Autodesk Inventor part; units mm, degrees
ref_plane "YZ Plane" through (0, 0, 0) normal (1, 0, 0) x (0, 1, 0)
ref_plane "XZ Plane" through (0, 0, 0) normal (0, 1, 0) x (-1, 0, 0)
ref_plane "XY Plane" through (0, 0, 0) normal (0, 0, 1) x (1, 0, 0)
sketch "Sketch1" plane through (0, 0, 0) normal (0, 0, 1) x (1, 0, 0)
  circle A0 centre (0, 0) radius 5
  line L0 (0, 7.8889) -> (6.832, 3.9445)
  line L1 (6.832, 3.9445) -> (6.832, -3.9445)
  line L2 (6.832, -3.9445) -> (0, -7.8889)
  line L3 (0, -7.8889) -> (-6.832, -3.9445)
  line L4 (-6.832, -3.9445) -> (-6.832, 3.9445)
  line L5 (-6.832, 3.9445) -> (0, 7.8889)
  dimension "d0" = 10
extrude "Extrusion1" add sketch "Sketch1" along normal blind 5.08
thread "Thread1"
properties part number "Nut"
Design review of the part built by this model. Coordinates are the model's own, in mm. Give positions to 0.01 mm unless a question says otherwise; leave off trailing zeros. Write each loop counter-clockwise with the first axis right and the second up, starting at its lowest first coordinate (ties: lowest second). Pieces come first, ordered by that corner, then holes. Notation, with made-up numbers: M 30,48 L 36,48 A8 ccw 36,53 Z; hole C 0.25,64.5 d9. An arc over 180 degrees is marked long. Answer as a JSON object with one key per item and string values. Group by question number.
1) We need section C-C (x = -2.5). Give the boundary of the cut face in (y, z).
2) We need section B-B (z = 4.4). Give the boundary of the cut face in (x, y).
3) Mouldability with a two-part tool opening along X and no side actions: class faces 1 (the face through (-0.1, -5.15, 5.08)), 2 (the face through (6.832, 0, 3)), 3 (the face through (-1.08, 4.88, 2.5)) as released by +X, released by -X, zero draft, split by the parting line, or undercut.
4) We need section A-A (y = 0.75). Give the boundary of the cut face in (x, z), and give its area (3 significant figures).
5) For line 1 along X through (y, z) = (3, 3.9); line 2 along Y through (x, z) = (-4, 2.1); line 3 along X through (y, z) = (4.25, 0.8), list the stretches that pass through material, from the lowest coordinate up.
6) We need section D-D (y = -6). Give the boundary of the cut face in (x, z), and give its area (3 significant figures).
7) Clearance check with flat-ended pins moving along their axes: pin 1 Ø2 at (x, z) = (-3, 4.5) entering from -Y; pin 2 Ø1.5 at (x, z) = (-4, 1) entering from -Y. State where each tip first meets the part, or that it passes through.
Answer key:
{
 "1": {"outline": "M -6.45,0 L -4.33,0 L -4.33,5.08 L -6.45,5.08 Z; M 4.33,0 L 6.45,0 L 6.45,5.08 L 4.33,5.08 Z"},
 "2": {"outline": "M -6.83,-3.94 L 0,-7.89 L 6.83,-3.94 L 6.83,3.94 L 0,7.89 L -6.83,3.94 Z; hole C 0,0 d10"},
 "3": {"face 1": "zero draft", "face 2": "released by +X", "face 3": "undercut"},
 "4": {"outline": "M -6.83,0 L -4.94,0 L -4.94,5.08 L -6.83,5.08 Z; M 4.94,0 L 6.83,0 L 6.83,5.08 L 4.94,5.08 Z", "area": "19.2 mm²"},
 "5": {"line 1": "x = -6.83 to -4, 4 to 6.83", "line 2": "y = -5.58 to -3, 3 to 5.58", "line 3": "x = -6.3 to -2.63, 2.63 to 6.3"},
 "6": {"outline": "M -3.27,0 L 3.27,0 L 3.27,5.08 L -3.27,5.08 Z", "area": "33.2 mm²"},
 "7": {"pin 1": "stops at y = -6.73", "pin 2": "stops at y = -6.01"}
}
